Verification items for the finished model (mm, model axes). Face numbers are marked on the shaded views. A direction names the side the tool comes from. Coordinates: 2 decimals unless noted, no trailing zeros. Order: outer loops, then holes, each group sorted by start corner. A loop starts at its lowest first (then second) coordinate and runs counter-clockwise, first axis right, second up. Notation, with made-up numbers: M -28.75,18.25 L -5.75,18.25 A24 ccw -5.75,28.25 Z; hole C -23.5,-13 d2. An arc over 180 degrees is marked long. Answer as a JSON object with one key per item and string values. Group by question number.
(1) Gauge pin test, flat ends, axial feed: pin 1 Ø1 at (x, z) = (35, -9) entering from -Y; pin 2 Ø5 at (x, y) = (68, -28.5) entering from -Z; pin 3 Ø1 at (x, y) = (42.5, -35.5) entering from -Z; pin 4 Ø1 at (x, y) = (43, 4.5) entering from -Z. Record the tip position at first contact, or that the pin passes through.
(2) Cross-section at B-B (z = 35.5). Enter the section's corners in (x, y), plus the area to 3 significant figures.
(3) Access from +Z, -Z, +X, -X, +Y, -Y to the whole of each face (thin tool, end or side, straight path). Record for the marked faces 1, 2 and 3.
(4) Cross-section at A-A (y = -44). Enter the section's corners in (x, z).
(5) Cross-section at D-D (y = 5). Enter the section's corners in (x, z).
(6) Cross-section at C-C (z = 23.4). Enter the section's corners in (x, y).
(7) Mould release check, pull along X, two halves, no side actions. Record for the marked faces 4, 5 and 6: released by +X, released by -X, zero draft, split by the parting line, or undercut.
(8) Material ranges on line 1 (X direction, y = -42, z = -1); line 2 (Z direction, x = 11, y = 5.75); line 3 (Z direction, x = 74.5, y = 6.25), recorded low to high.
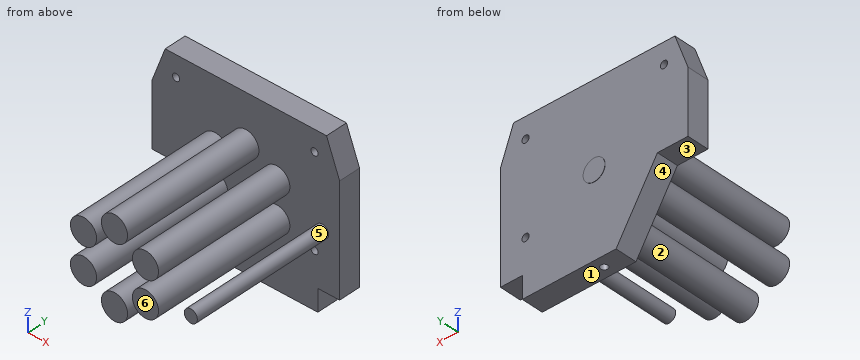
from build123d import *

# Parameters (mm, degrees)
BOSS_EXTRUDE1_DEPTH = 10
CHAMFER1_SIZE       = 6
CHAMFER1_SIZE2      = 16
CHAMFER2_SIZE       = 16
CHAMFER2_SIZE2      = 6
SKETCH2_W           = 10
SKETCH2_H           = 10
CUT_EXTRUDE1_DEPTH  = 10
BOSS_EXTRUDE2_DEPTH = 0.1
SKETCH4_R           = 6
BOSS_EXTRUDE3_DEPTH = 76
SKETCH5_R           = 3
BOSS_EXTRUDE4_DEPTH = 76
SKETCH6_R           = 1.65
CUT_EXTRUDE2_DEPTH  = 11.1
SKETCH7_R           = 1.65
CUT_EXTRUDE3_DEPTH  = 10


with BuildPart() as part:
    # Sketch1 → Boss-Extrude1 (new body)
    with BuildSketch(Plane(origin=(0, 0, 0), x_dir=(1, 0, 0), z_dir=(0, 1, 0))):
        Polygon((0, 0), (0, -45), (86, -45), (86, 31), (33, 31), (14, 0), align=None)
    extrude(amount=BOSS_EXTRUDE1_DEPTH)

    # Chamfer1
    chamfer1_edges = [part.edges().sort_by_distance(p)[0] for p in [
        (86, 5, 45),
    ]]
    chamfer1_side = [part.faces().sort_by_distance(p)[0] for p in [
        (43, 5, 45),
    ]]
    chamfer(chamfer1_edges, length=CHAMFER1_SIZE, length2=CHAMFER1_SIZE2, reference=chamfer1_side[0])

    # Chamfer2
    chamfer2_edges = [part.edges().sort_by_distance(p)[0] for p in [
        (0, 5, 45),
    ]]
    chamfer2_side = [part.faces().sort_by_distance(p)[0] for p in [
        (0, 5, 22.5),
    ]]
    chamfer(chamfer2_edges, length=CHAMFER2_SIZE, length2=CHAMFER2_SIZE2, reference=chamfer2_side[0])

    # Sketch2 → Cut-Extrude1 (cut)
    with BuildSketch(Plane(origin=(0, 10, 0), x_dir=(1, 0, 0), z_dir=(0, 1, 0))):
        with Locations((81, 26)):
            Rectangle(SKETCH2_W, SKETCH2_H)
    extrude(amount=-CUT_EXTRUDE1_DEPTH, mode=Mode.SUBTRACT)

    # Sketch3 → Boss-Extrude2 (add)
    with BuildSketch(Plane(origin=(0, 10, 0), x_dir=(1, 0, 0), z_dir=(0, 1, 0))):
        with BuildLine():
            ThreePointArc((41.3, -2.297872822), (43, -12), (44.7, -2.297872822))
            ThreePointArc((44.7, -2.297872822), (43, -2), (41.3, -2.297872822))
        make_face()
    extrude(amount=BOSS_EXTRUDE2_DEPTH)

    # Sketch4 → Boss-Extrude3 (add)
    with BuildSketch(Plane(origin=(0, 10, 0), x_dir=(1, 0, 0), z_dir=(0, 1, 0))):
        with Locations((43, 9.4)):
            Circle(SKETCH4_R)
        with Locations((57.202816622, 1.2)):
            Circle(SKETCH4_R)
        with Locations((57.202816622, -15.2)):
            Circle(SKETCH4_R)
        with Locations((43, -23.4)):
            Circle(SKETCH4_R)
        with Locations((28.797183378, -15.2)):
            Circle(SKETCH4_R)
        with Locations((28.797183378, 1.2)):
            Circle(SKETCH4_R)
    extrude(amount=-BOSS_EXTRUDE3_DEPTH)

    # Sketch5 → Boss-Extrude4 (add)
    with BuildSketch(Plane(origin=(0, 10, 0), x_dir=(1, 0, 0), z_dir=(0, 1, 0))):
        with Locations((78, -4)):
            Circle(SKETCH5_R)
    extrude(amount=-BOSS_EXTRUDE4_DEPTH)

    # Sketch6 → Cut-Extrude2 (cut, through all)
    with BuildSketch(Plane.XZ):
        with Locations((74.5, -5.8)):
            Circle(SKETCH6_R)
        with Locations((74.5, 35.5)):
            Circle(SKETCH6_R)
        with Locations((11, 35.5)):
            Circle(SKETCH6_R)
    extrude(amount=-CUT_EXTRUDE2_DEPTH, mode=Mode.SUBTRACT)

    # Sketch7 → Cut-Extrude3 (cut)
    with BuildSketch(Plane(origin=(0, 0, -31), x_dir=(-1, 0, 0), z_dir=(0, 0, -1))):
        with Locations((-43, 5)):
            Circle(SKETCH7_R)
    extrude(amount=-CUT_EXTRUDE3_DEPTH, mode=Mode.SUBTRACT)


solid = part.part
Taken from the geometry:
{
 "1": {"pin 1": "stops at y = 0", "pin 2": "passes through", "pin 3": "stops at z = -15.4", "pin 4": "stops at z = -21"},
 "2": {"outline": "M 2.44,0 L 9.35,0 L 9.35,10 L 2.44,10 Z; M 12.65,0 L 72.85,0 L 72.85,10 L 12.65,10 Z; M 76.15,0 L 83.56,0 L 83.56,10 L 76.15,10 Z", "area": "745 mm²"},
 "3": {"face 1": "-Z, +X, -X, +Y, -Y", "face 2": "-Y", "face 3": "-Z, -X, +Y, -Y"},
 "4": {"outline": "C 28.8,-1.2 d12; C 28.8,15.2 d12; C 43,-9.4 d12; C 43,23.4 d12; C 57.2,-1.2 d12; C 57.2,15.2 d12; C 78,4 d6"},
 "5": {"outline": "M 0,0 L 14,0 L 33,-31 L 41.35,-31 L 41.35,-21 L 44.65,-21 L 44.65,-31 L 76,-31 L 76,-21 L 86,-21 L 86,29 L 80,45 L 6,45 L 0,29 Z; hole C 11,35.5 d3.3; hole C 74.5,-5.8 d3.3; hole C 74.5,35.5 d3.3"},
 "6": {"outline": "M 0,0 L 37,0 L 37,-66 L 49,-66 L 49,0 L 86,0 L 86,10 L 0,10 Z"},
 "7": {"face 4": "released by -X", "face 5": "undercut", "face 6": "zero draft"},
 "8": {"line 1": "x = 22.8 to 34.79, 51.21 to 63.2", "line 2": "z = 0 to 33.85, 37.15 to 45", "line 3": "z = -31 to -7.45, -4.15 to 33.85, 37.15 to 45"}
}
